The listing builds one solid part. Answer for the finished solid, in the listing's coordinates (mm). Face numbers are marked on the shaded views. A direction names the side the tool comes from. Give positions to 0.01 mm unless a question says otherwise; leave off trailing zeros. Write each loop counter-clockwise with the first axis right and the second up, starting at its lowest first coordinate (ties: lowest second). Pieces come first, ordered by that corner, then holes. Notation, with made-up numbers: (67, 48) - (78, 48) arc R19 cw to (78, 72) - close; hole circle Ø10 at (8, 64). An arc over 180 degrees is marked (long way). Return JSON: item names as keys, results as strings.
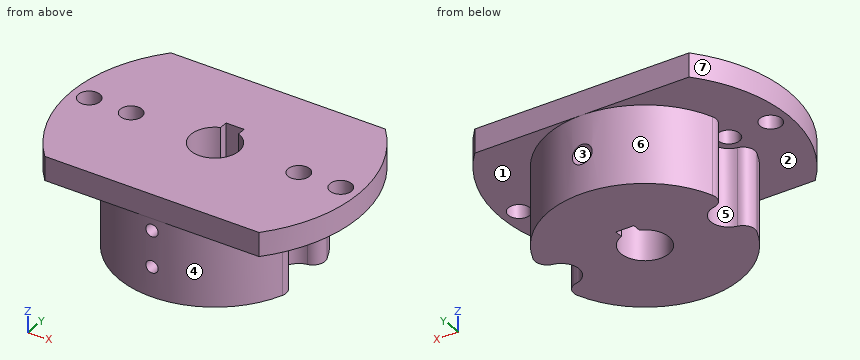
from build123d import *

# Parameters (mm, degrees)
BOSS_EXTRUDE1_DEPTH          = 4
BOSS_EXTRUDE2_REACH          = 35.481
M3_CLEARANCE_HOLE1_D         = 3.6
F_8_0MM_DOWEL_HOLE1_D        = 8
FILLET1_R                    = 2
M4X0_7_TAPPED_HOLE1_REACH    = 45.081
M4X0_7_TAPPED_HOLE1_BORE_R   = 1.65
M2_5X0_45_TAPPED_HOLE1_D     = 2.05
M2_5X0_45_TAPPED_HOLE1_DEPTH = 8
M2_5X0_45_TAPPED_HOLE1_TIP   = 0.615882135
SKETCH14_W                   = 3
SKETCH14_H                   = 3
CUT_EXTRUDE1_DEPTH           = 34.481338272


with BuildPart() as part:
    # Sketch1 → Boss-Extrude1 (new body)
    with BuildSketch(Plane(origin=(0, 0, 12), x_dir=(-1, 0, 0), z_dir=(0, 0, -1))):
        with BuildLine():
            Line((17.88854382, 16), (-17.88854382, 16))
            ThreePointArc((-17.88854382, 16), (-24, 0), (-17.88854382, -16))
            Line((-17.88854382, -16), (17.88854382, -16))
            ThreePointArc((17.88854382, -16), (24, 0), (17.88854382, 16))
        make_face()
    extrude(amount=-BOSS_EXTRUDE1_DEPTH)

    # Sketch3 → Boss-Extrude2 (add, up to next)
    with BuildSketch(Plane(origin=(0, 0, -1), x_dir=(-1, 0, 0), z_dir=(0, 0, -1)), mode=Mode.PRIVATE) as boss_extrude2_sk1:
        with BuildLine():
            ThreePointArc((-15.821428571, -2.383778085), (0, -16), (15.821428571, -2.383778085))
            ThreePointArc((15.821428571, -2.383778085), (11, 0), (15.821428571, 2.383778085))
            ThreePointArc((15.821428571, 2.383778085), (0, 16), (-15.821428571, 2.383778085))
            ThreePointArc((-15.821428571, 2.383778085), (-11, 0), (-15.821428571, -2.383778085))
        make_face()
    boss_extrude2_tool1 = extrude(boss_extrude2_sk1.sketch, amount=-BOSS_EXTRUDE2_REACH, mode=Mode.PRIVATE) - part.part
    add(boss_extrude2_tool1.solids().sort_by_distance((0, 0, -1))[0])

    # M3 Clearance Hole1 (through all)
    with Locations(Plane(origin=(0, 0, 12), x_dir=(-1, 0, 0), z_dir=(0, 0, -1))):
        with Locations((21, 0), (-21, 0), (-14, 0), (14, 0)):
            Hole(M3_CLEARANCE_HOLE1_D / 2)

    # Ø8.0mm Dowel Hole1 (through all)
    with Locations(Plane(origin=(0, 0, -1), x_dir=(-1, 0, 0), z_dir=(0, 0, -1))):
        with Locations((0, 0)):
            Hole(F_8_0MM_DOWEL_HOLE1_D / 2)

    # Fillet1
    fillet1_edges = [part.edges().sort_by_distance(p)[0] for p in [
        (-15.821428571, -2.383778085, 5.5),
        (-15.821428571, 2.383778085, 5.5),
        (15.821428571, 2.383778085, 5.5),
        (15.821428571, -2.383778085, 5.5),
    ]]
    fillet(fillet1_edges, radius=FILLET1_R)

    # M4x0.7 Tapped Hole1 bore → M4x0.7 Tapped Hole1 (cut, up to next)
    with BuildSketch(Plane(origin=(0, 16, 0), x_dir=(1, 0, 0), z_dir=(0, 1, 0)), mode=Mode.PRIVATE) as m4x0_7_tapped_hole1_sk1:
        with Locations((0, -5.5)):
            Circle(M4X0_7_TAPPED_HOLE1_BORE_R)
    m4x0_7_tapped_hole1_tool1 = extrude(m4x0_7_tapped_hole1_sk1.sketch, amount=-M4X0_7_TAPPED_HOLE1_REACH, mode=Mode.PRIVATE) & part.part
    add(m4x0_7_tapped_hole1_tool1.solids().sort_by_distance((0, 16, 5.5))[0], mode=Mode.SUBTRACT)

    # M2.5x0.45 Tapped Hole1
    with Locations(Plane(origin=(0, -16, 0), x_dir=(-1, 0, 0), z_dir=(0, -1, 0))):
        with Locations((0, -4), (0, -10)):
            Hole(M2_5X0_45_TAPPED_HOLE1_D / 2, depth=M2_5X0_45_TAPPED_HOLE1_DEPTH)
            with Locations((0, 0, -(M2_5X0_45_TAPPED_HOLE1_DEPTH + M2_5X0_45_TAPPED_HOLE1_TIP / 2))):  # 118° drill point
                Cone(0, M2_5X0_45_TAPPED_HOLE1_D / 2, M2_5X0_45_TAPPED_HOLE1_TIP, mode=Mode.SUBTRACT)

    # Sketch14 → Cut-Extrude1 (cut, through all)
    with BuildSketch(Plane(origin=(0, 0, -1), x_dir=(-1, 0, 0), z_dir=(0, 0, -1))):
        with Locations((0, 3.6)):
            Rectangle(SKETCH14_W, SKETCH14_H)
    extrude(amount=-CUT_EXTRUDE1_DEPTH, mode=Mode.SUBTRACT)


solid = part.part
Item 1: For the marked faces 1, 2, 3 and 4, determine the directions among +Z, -Z, +X, -X, +Y, -Y from which every point of the face is accessible in a straight line to the end or side of a thin tool.
Answer below:
{"face 1": "-Z, +X", "face 2": "-Z, -X", "face 3": "+Y", "face 4": "-Z, -Y"}
Item 2: A cutting plane is placed at C-C on y = -12. Determine the outline of the cut face in (x, z) (3 decimals).
Answer below:
{"outline": "(-20.785, 12) - (-10.583, 12) - (-10.583, -1) - (10.583, -1) - (10.583, 12) - (20.785, 12) - (20.785, 16) - (-20.785, 16) - close; hole circle Ø2.05 at (0, 4); hole circle Ø2.05 at (0, 10)"}
Item 3: A cutting plane is placed at A-A on z = 14.75. Determine the outline of the cut face in (x, y).
Answer below:
{"outline": "(-17.89, -16) - (17.89, -16) arc R24 ccw to (17.89, 16) - (-17.89, 16) arc R24 ccw to start; hole circle Ø3.6 at (-21, 0); hole circle Ø3.6 at (-14, 0); hole (-1.5, 3.71) arc R4 ccw (long way) to (1.5, 3.71) - (1.5, 5.1) - (-1.5, 5.1) - close; hole circle Ø3.6 at (14, 0); hole circle Ø3.6 at (21, 0)"}
Item 4: The mould has two halves that part along Y. Classify the marked faces 5, 6 and 7: +Y half, -Y half, draft (parallel to the pull), parting line (faces both ways), or undercut.
Answer below:
{"face 5": "undercut", "face 6": "+Y half", "face 7": "parting line"}
Item 5: A cutting plane is placed at B-B on x = 3. Determine the outline of the cut face in (y, z), then the cut area to 3 significant figures.
Answer below:
{"outline": "(-16, 12) - (-15.72, 12) - (-15.72, -1) - (-2.65, -1) - (-2.65, 16) - (-16, 16) - close; (2.65, -1) - (15.72, -1) - (15.72, 12) - (16, 12) - (16, 16) - (2.65, 16) - close", "area": "447 mm²"}
Item 6: Consider L1, parallel to Z at x = 0, y = -10 (3 decimals); L2, parallel to Z at x = 0, y = 11; L3, parallel to X at y = 0, z = 4. Determine where each line is inside the solid, lowest interval first.
Answer below:
{"L1": "z = -1 to 2.975, 5.025 to 8.975, 11.025 to 16", "L2": "z = -1 to 3.85, 7.15 to 16", "L3": "x = -11 to -4, 4 to 11"}
Item 7: A cutting plane is placed at D-D on y = 9. Determine the outline of the cut face in (x, z), then the cut area to 3 significant figures.
Answer below:
{"outline": "(-22.25, 12) - (-13.23, 12) - (-13.23, -1) - (13.23, -1) - (13.23, 12) - (22.25, 12) - (22.25, 16) - (-22.25, 16) - close; hole circle Ø3.3 at (0, 5.5)", "area": "513 mm²"}
Item 8: Flat-ended cylindrical pins translate along their axes: P1, Ø3, axis at x = 14, y = 0, coming from the +Z side; P2, Ø1.6, axis at x = 0, z = 10, coming from the -Y side; P3, Ø2, axis at x = -10, z = 4, coming from the +Y side; P4, Ø0.7, axis at y = 4, z = 3, coming from the +X side. Find the tip coordinate at first contact, or state that the pin passes through.
Answer below:
{"P1": "passes through", "P2": "stops at y = -7.86", "P3": "stops at y = 13.23", "P4": "stops at x = 15.02"}
